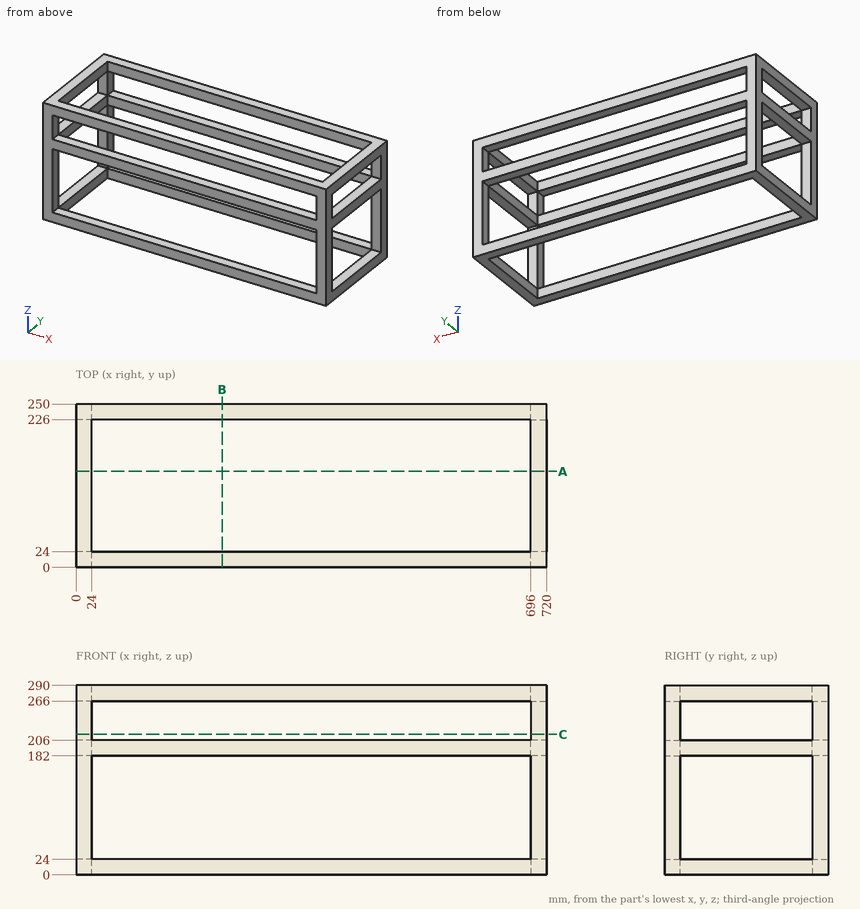
Check sheet for the drawn part. Datum: minimum x, y, z corner. Units: mm. Give positions to 0.01 mm unless a question says otherwise; leave off trailing zeros. Order: outer loops, then holes, each group sorted by start corner. A loop starts at its lowest first (then second) coordinate and runs counter-clockwise, first axis right, second up. Notation, with made-up numbers: (29.25, -27.5) - (84.25, -27.5) arc R6 ccw to (84.25, -20.5) - close; hole circle Ø1 at (82.5, 66.5). An arc over 180 degrees is marked (long way). Answer in a Markdown table with one row per item. Add a question column.
Q1. Material ranges on probe 1 along Z at (x, y) = (160, 15); probe 2 along Y at (x, z) = (205.5, 201.5); probe 3 along X at (y, z) = (78, 203), recorded low to high. Write a range as from..to.
Q2. Cross-section at C-C, the plane z = 215. Enter the section's corners in (x, y), then the cut area to 3 significant figures.
Q3. Cross-section at B-B, the plane x = 223.5. Enter the section's corners in (y, z).
Q4. Cross-section at A-A, the plane y = 147. Enter the section's corners in (x, z).
Check values:
| question | item | result |
|---|---|---|
| 1 | probe 1 | z = 0..24, 182..206, 266..290 |
| 1 | probe 2 | y = 0..24, 226..250 |
| 1 | probe 3 | x = 0..24, 696..720 |
| 2 | outline | (0, 0) - (24, 0) - (24, 24) - (0, 24) - close; (0, 226) - (24, 226) - (24, 250) - (0, 250) - close; (696, 0) - (720, 0) - (720, 24) - (696, 24) - close; (696, 226) - (720, 226) - (720, 250) - (696, 250) - close |
| 2 | area | 2,300 mm^2 |
| 3 | outline | (0, 0) - (24, 0) - (24, 24) - (0, 24) - close; (0, 182) - (24, 182) - (24, 206) - (0, 206) - close; (0, 266) - (24, 266) - (24, 290) - (0, 290) - close; (226, 0) - (250, 0) - (250, 24) - (226, 24) - close; (226, 182) - (250, 182) - (250, 206) - (226, 206) - close; (226, 266) - (250, 266) - (250, 290) - (226, 290) - close |
| 4 | outline | (0, 0) - (24, 0) - (24, 24) - (0, 24) - close; (0, 182) - (24, 182) - (24, 206) - (0, 206) - close; (0, 266) - (24, 266) - (24, 290) - (0, 290) - close; (696, 0) - (720, 0) - (720, 24) - (696, 24) - close; (696, 182) - (720, 182) - (720, 206) - (696, 206) - close; (696, 266) - (720, 266) - (720, 290) - (696, 290) - close |
